Design review of the part built by this model. Coordinates are the model's own, in mm. Give positions to 0.01 mm unless a question says otherwise; leave off trailing zeros. Order: outer loops, then holes, each group sorted by start corner. A loop starts at its lowest first (then second) coordinate and runs counter-clockwise, first axis right, second up. Notation, with made-up numbers: (55, 69.5) -> (86, 69.5) arc R20 cw to (86, 106.5) -> close; hole circle Ø5 at (18, 38.25). An arc over 180 degrees is marked (long way). Return JSON: item names as keys, results as strings.
```python
from build123d import *

# Parameters (mm, degrees)
SKETCH7_R                = 4
SKETCH7_R_2              = 2
BOSS_EXTRUDE1_DEPTH      = 5
HOLE_WIZARD_M3_5_1_D     = 3.9
HOLE_WIZARD_M3_5_1_DEPTH = 10
HOLE_WIZARD_M3_5_1_TIP   = 1.171678207
SKETCH_4_R               = 1.75
CUT_EXTRUDE_1_DEPTH      = 10
EXTRUDE_START            = 5
SKETCH_5_R               = 17.5
SKETCH_5_R_2             = 1.75
SKETCH_5_R_3             = 4
EXTRUDE_1_DEPTH          = 5


with BuildPart() as part:
    # Sketch7 → Boss-Extrude1 (new body)
    with BuildSketch(Plane.XY):
        with BuildLine():
            Line((8.994200014, 237.123057432), (17.48872225, 0.62816723))
            ThreePointArc((17.48872225, 0.62816723), (0, -17.5), (-17.48872225, 0.62816723))
            Line((-17.48872225, 0.62816723), (-8.994200014, 237.123057432))
            ThreePointArc((-8.994200014, 237.123057432), (0, 245.8), (8.994200014, 237.123057432))
        make_face()
        Circle(SKETCH7_R, mode=Mode.SUBTRACT)
        with Locations((0, 236.8)):
            Circle(SKETCH7_R_2, mode=Mode.SUBTRACT)
    extrude(amount=-BOSS_EXTRUDE1_DEPTH)

    # M3.5 间隙孔1
    with Locations(Plane(origin=(0, 156.8, 0), x_dir=(1, 0, 0), z_dir=(0, 0, 1))):
        with Locations((0, 0), (0, -76.8)):
            Hole(HOLE_WIZARD_M3_5_1_D / 2, depth=HOLE_WIZARD_M3_5_1_DEPTH)
            with Locations((0, 0, -(HOLE_WIZARD_M3_5_1_DEPTH + HOLE_WIZARD_M3_5_1_TIP / 2))):  # 118° drill point
                Cone(0, HOLE_WIZARD_M3_5_1_D / 2, HOLE_WIZARD_M3_5_1_TIP, mode=Mode.SUBTRACT)

    # 草图4 → 切除-拉伸1 (cut)
    with BuildSketch(Plane.XY):
        with Locations((7, 0)):
            Circle(SKETCH_4_R)
        with Locations((0, 7)):
            Circle(SKETCH_4_R)
        with Locations((0, -7)):
            Circle(SKETCH_4_R)
        with Locations((-7, 0)):
            Circle(SKETCH_4_R)
    extrude(amount=-CUT_EXTRUDE_1_DEPTH, mode=Mode.SUBTRACT)

    # 草图5 → 凸台-拉伸1 (add)
    with BuildSketch(Plane.XY.offset(EXTRUDE_START)):
        Circle(SKETCH_5_R)
        with Locations((7, 0)):
            Circle(SKETCH_5_R_2, mode=Mode.SUBTRACT)
        with Locations((0, -7)):
            Circle(SKETCH_5_R_2, mode=Mode.SUBTRACT)
        Circle(SKETCH_5_R_3, mode=Mode.SUBTRACT)
        with Locations((-7, 0)):
            Circle(SKETCH_5_R_2, mode=Mode.SUBTRACT)
        with Locations((0, 7)):
            Circle(SKETCH_5_R_2, mode=Mode.SUBTRACT)
    extrude(amount=-EXTRUDE_1_DEPTH)


solid = part.part
```
Item 1: Add section C-C (y = 34.5). Give the boundary of the cut face in (x, z), plus the area to 3 significant figures.
Result set:
{"outline": "(-16.27, -5) -> (16.27, -5) -> (16.27, 0) -> (-16.27, 0) -> close", "area": "163 mm^2"}
Item 2: Wall thickness on L1, parallel to Y at x = 0, z = 2; L2, parallel to Z at x = -2, y = 36.5; L3, parallel to Y at x = 3, z = -4.5: over which ranges is each line inside the solid? List them lowest first. Write a range as [from, to].
Result set:
{"L1": "y = [-17.5, -8.75], [-5.25, -4], [4, 5.25], [8.75, 17.5]", "L2": "z = [-5, 0]", "L3": "y = [-17.24, -2.65], [2.65, 245.29]"}
Item 3: Add section A-A (z = -2.75). Give the number of separate pieces and of enclosed holes in the cut face, plus the area to 3 significant figures.
Result set:
{"separate pieces": "1", "enclosed holes": "8", "area": "6,760 mm^2"}
Item 4: Mouldability with a two-part tool opening along X and no side actions: class faces 1 (the face through (-0.193, 245.798, -2.465)), 2 (the face through (-0.867, -3.905, 0.07)), 3 (the face through (0, 116, -5)) as released by +X, released by -X, zero draft, split by the parting line, or undercut.
Result set:
{"face 1": "split by the parting line", "face 2": "undercut", "face 3": "zero draft"}
Item 5: Add section B-B (y = 104.5). Give the boundary of the cut face in (x, z), plus the area to 3 significant figures.
Result set:
{"outline": "(-13.76, -5) -> (13.76, -5) -> (13.76, 0) -> (-13.76, 0) -> close", "area": "138 mm^2"}
Item 6: For pin 1 (17.5 mm diameter, centred on x = 6.5, y = 140.5, fed in from +Z); pin 2 (1.5 mm diameter, centred on x = 13, z = -3.5, fed in from -Y); pin 3 (1.5 mm diameter, centred on y = 37, z = 0, fed in from +X), all flat-tipped, find the tip position at first contact; note any pin that passes through.
Result set:
{"pin 1": "stops at z = 0", "pin 2": "stops at y = -12.5", "pin 3": "stops at x = 16.21"}
